```python
from build123d import *

# Parameters (mm, degrees)
SKETCH1_R           = 12.5
BOSS_EXTRUDE1_DEPTH = 2.5
SKETCH4_W           = 4
SKETCH4_H           = 27.5
BOSS_EXTRUDE3_DEPTH = 5
CIRPATTERN7_COUNT   = 4
CUT_EXTRUDE3_REACH  = 41.211
SKETCH8_W           = 12.6
SKETCH8_H           = 12.5
FILLET1_R           = 1


with BuildPart() as part:
    # Sketch1 → Boss-Extrude1 (new, symmetric)
    with BuildSketch(Plane.XY):
        Circle(SKETCH1_R)
    extrude(amount=BOSS_EXTRUDE1_DEPTH, both=True)

    # Sketch4 → Boss-Extrude3 (add)
    with BuildSketch(Plane.XY.offset(2.5)):
        with Locations((-7, 13.75)):
            Rectangle(SKETCH4_W, SKETCH4_H)
        with Locations((7, 13.75)):
            Rectangle(SKETCH4_W, SKETCH4_H)
    boss_extrude3 = extrude(amount=-BOSS_EXTRUDE3_DEPTH)

    # CirPattern7: Boss-Extrude3 ×4 about axis
    cirpattern7_axis = Axis((0, 0, 0), (0, 0, 1))
    for i in range(1, CIRPATTERN7_COUNT):
        add(boss_extrude3.rotate(cirpattern7_axis, i * 360 / CIRPATTERN7_COUNT))

    # Sketch8 → Cut-Extrude3 (cut, up to next)
    with BuildSketch(Plane.XY.offset(2.5), mode=Mode.PRIVATE) as cut_extrude3_sk1:
        Rectangle(SKETCH8_W, SKETCH8_H)
    cut_extrude3_tool1 = extrude(cut_extrude3_sk1.sketch, amount=-CUT_EXTRUDE3_REACH, mode=Mode.PRIVATE) & part.part
    add(cut_extrude3_tool1.solids().sort_by_distance((0, 0, 2.5))[0], mode=Mode.SUBTRACT)

    # Fillet1
    fillet1_edges = [part.edges().sort_by_distance(p)[0] for p in [
        (6.3, 6.25, 0),
        (6.3, -6.25, 0),
        (-6.3, -6.25, 0),
        (-6.3, 6.25, 0),
    ]]
    fillet(fillet1_edges, radius=FILLET1_R)


solid = part.part
```
Part model, mm, in its own coordinate system. A direction names the side the tool comes from. Coordinates: 2 decimals unless noted, no trailing zeros. Loops run counter-clockwise (first coordinate to the right, second up) from the corner with the lowest first, then second, coordinate; pieces in that order, holes last. Notation, with made-up numbers: (-38, -31.5) - (3, -31.5) arc R20 ccw to (3, -27.5) - close; hole circle Ø1 at (-34.75, -11). An arc over 180 degrees is marked (long way). Write item = value, one per line. Start each with the question number.
Item 1: 3-axis set-ups, long thin cutter, end or side, ignore diameter. For faces 4 (the flat face through (-19, 5, 0)), 5 (the flat face through (18, 9, 0)), 6 (the flat face through (-9, 18, 0)), 7 (the flat face through (9, -18, 0)), 8 (the flat face through (5, -19, 0)): which of +Z, -Z, +X, -X, +Y, -Y reach the whole face in a straight line?
Item 2: Mould opens along Y. For faces 1 (the flat face through (0, -6.25, 0)), 2 (the flat face through (27.5, 7, 0)), 3 (the flat face through (-18, -9, 0)) say: released by +Y, released by -Y, zero draft, split by the parting line, or undercut.
Item 3: Cut at C-C, the plane x = 10. Give the cut face in (y, z).
Item 4: Cut at A-A, the plane y = 21. Give the cut face in (x, z), and give its area (3 significant figures).
Item 5: Wall check: L1, parallel to Y at x = 18.5, z = 0.3; L2, parallel to Y at x = 10, z = -1.8. Give the ranges that are in metal, low to high. Write a range as from..to.
Item 6: Flat gauge pins, fed straight in: pin 1 Ø2.5 at (x, z) = (-0.5, 0) entering from +Y; pin 2 Ø1 at (x, z) = (-10, -1) entering from -Y; pin 3 Ø3 at (y, z) = (13.5, -2) entering from -X. Where does each tip first touch, or does it go through?
The answers:
q1.face_4 = +Z, -Z, -X
q1.face_5 = +Z, -Z, +X, +Y
q1.face_6 = +Z, -Z, -X, +Y
q1.face_7 = +Z, -Z, +X, -Y
q1.face_8 = +Z, -Z, -Y
q2.face_1 = undercut
q2.face_2 = zero draft
q2.face_3 = released by -Y
q3.outline = (-9, -2.5) - (9, -2.5) - (9, 2.5) - (-9, 2.5) - close
q4.outline = (-9, -2.5) - (-5, -2.5) - (-5, 2.5) - (-9, 2.5) - close; (5, -2.5) - (9, -2.5) - (9, 2.5) - (5, 2.5) - close
q4.area = 40.0 mm2
q5.L1 = -9..-5, 5..9
q5.L2 = -9..9
q6.pin_1 = 12.5
q6.pin_2 = -9
q6.pin_3 = -9
